Could you check a few things on this model? Use its own coordinates, in mm. A direction names the side the tool comes from. Coordinates: 2 decimals unless noted, no trailing zeros. Order: outer loops, then holes, each group sorted by start corner. A loop starts at its lowest first (then second) coordinate and runs counter-clockwise, first axis right, second up. Notation, with made-up numbers: (68.5, 66.5) - (91.5, 66.5) arc R13 cw to (91.5, 74.5) - close; hole circle Ø11 at (26, 36.5). An arc over 180 degrees is marked (long way). Answer as a JSON object with one key per item and string values. Group by question number.
(1) Imagine slicing it at B-B, the plane y = 31. Write out the boundary of the cut face in (x, z), and give its area (3 significant figures).
(2) Imagine slicing it at D-D, the plane z = 12. Write out the boundary of the cut face in (x, y).
(3) We'd pull the mould along Z, two halves only. Please class faces 1 (the cylindrical face through (-13.91, 24.65, -3.09)), 2 (the cylindrical face through (12.53, 23.17, 1.64)), 3 (the flat face through (0, 62, 0)): pulls with the +Z half, pulls with the -Z half, needs draft (parallel to the pull), parting line crosses it, or undercut.
(4) Which directions (+Z, -Z, +X, -X, +Y, -Y) give clear straight access to the entire face, cutting with the end or side of a thin tool? Please do faces 4 (the flat face through (3.4, 50, 6.1)), 5 (the flat face through (0, 47, 0)), 6 (the flat face through (-13, 0, -1)).
(5) Will these pins go through, and if not, where does the flat tip stop? P1, Ø1, axis at x = -2, z = -7, coming from the +Y side; P2, Ø3, axis at y = 12.5, z = -2, coming from the -X side; P3, Ø10, axis at x = 2, y = 21, coming from the +Z side; P4, Ø3, axis at x = -1, z = -10, coming from the -Y side.
(6) Imagine slicing it at C-C, the plane x = 0. Write out the boundary of the cut face in (y, z), and give its area (3 significant figures).
(7) Imagine slicing it at A-A, the plane z = 0. Write out the boundary of the cut face in (x, y), and give its area (3 significant figures).
(8) Please list where these lines run through material, in increasing order: probe 1 along X at (y, z) = (17, 0); probe 2 along Y at (x, z) = (-3.75, -11.5); probe 3 along X at (y, z) = (33, 9.5).
from build123d import *

# Parameters (mm, degrees)
IZIM3_R                     = 14.25
Y_KSEKLIK_EKSTR_ZYON2_DEPTH = 50
IZIM4_R                     = 3.75
Y_KSEKLIK_EKSTR_ZYON3_DEPTH = 12
RADYUS1_R                   = 3
RADYUS2_R                   = 1
IZIM5_R                     = 12.635430767
KES_EKSTR_ZYON1_DEPTH       = 47


with BuildPart() as part:
    # Çizim3 → Yükseklik-Ekstrüzyon2 (new body)
    with BuildSketch(Plane(origin=(0, 0, 0), x_dir=(1, 0, 0), z_dir=(0, 1, 0))):
        with Locations(Location((0, 0, 0), (0, 0, 270))):
            Circle(IZIM3_R)
    extrude(amount=Y_KSEKLIK_EKSTR_ZYON2_DEPTH)

    # Çizim4 → Yükseklik-Ekstrüzyon3 (add)
    with BuildSketch(Plane(origin=(0, 50, 0), x_dir=(1, 0, 0), z_dir=(0, 1, 0))):
        with Locations(Location((0, 0, 0), (0, 0, 270))):
            Circle(IZIM4_R)
    extrude(amount=Y_KSEKLIK_EKSTR_ZYON3_DEPTH)

    # Radyus1
    radyus1_edges = [part.edges().sort_by_distance(p)[0] for p in [
        (0, 50, -3.75),
    ]]
    fillet(radyus1_edges, radius=RADYUS1_R)

    # Radyus2
    radyus2_edges = [part.edges().sort_by_distance(p)[0] for p in [
        (0, 62, -3.75),
    ]]
    fillet(radyus2_edges, radius=RADYUS2_R)

    # Çizim5 → Kes-Ekstrüzyon1 (cut)
    with BuildSketch(Plane.XZ):
        with Locations(Location((0, 0, 0), (0, 0, 270))):
            Circle(IZIM5_R)
    extrude(amount=-KES_EKSTR_ZYON1_DEPTH, mode=Mode.SUBTRACT)


solid = part.part
Result set:
{
 "1": {"outline": "circle Ø28.5 at (0, 0); hole circle Ø25.27 at (0, 0)", "area": "136 mm^2"},
 "2": {"outline": "(-7.69, 0) - (-3.96, 0) - (-3.96, 47) - (3.96, 47) - (3.96, 0) - (7.69, 0) - (7.69, 50) - (-7.69, 50) - close"},
 "3": {"face 1": "parting line crosses it", "face 2": "undercut", "face 3": "needs draft"},
 "4": {"face 4": "+Y", "face 5": "-Y", "face 6": "+Z, -Z, +X, -X, -Y"},
 "5": {"P1": "stops at y = 50", "P2": "stops at x = -14.24", "P3": "stops at z = 14.25", "P4": "stops at y = 47"},
 "6": {"outline": "(0, -14.25) - (50, -14.25) - (50, -6.75) arc R3 cw to (53, -3.75) - (61, -3.75) arc R1 ccw to (62, -2.75) - (62, 2.75) arc R1 ccw to (61, 3.75) - (53, 3.75) arc R3 cw to (50, 6.75) - (50, 14.25) - (0, 14.25) - (0, 12.64) - (47, 12.64) - (47, -12.64) - (0, -12.64) - close", "area": "331 mm^2"},
 "7": {"outline": "(-14.25, 0) - (-12.64, 0) - (-12.64, 47) - (12.64, 47) - (12.64, 0) - (14.25, 0) - (14.25, 50) - (6.75, 50) arc R3 cw to (3.75, 53) - (3.75, 61) arc R1 ccw to (2.75, 62) - (-2.75, 62) arc R1 ccw to (-3.75, 61) - (-3.75, 53) arc R3 cw to (-6.75, 50) - (-14.25, 50) - close", "area": "331 mm^2"},
 "8": {"probe 1": "x = -14.25 to -12.64, 12.64 to 14.25", "probe 2": "y = 47 to 50", "probe 3": "x = -10.62 to -8.33, 8.33 to 10.62"}
}
